```python
from build123d import *

# Parameters (mm, degrees)
F1_DEPTH = 40.2336
F0_R     = 10.16
F2_DEPTH = 15.7734
F3_SIZE  = 3.302


with BuildPart() as f1:
    # F0 (on Top) → F1 (new body)
    with BuildSketch(Plane.XY):
        with BuildLine():
            ThreePointArc((5.050141, -28.125197), (21.918467, -18.333342), (28.575, 0))
            ThreePointArc((28.575, 0), (21.918467, 18.333342), (5.050141, 28.125197))
            ThreePointArc((5.050141, 28.125197), (-28.575, 0), (5.050141, -28.125197))
        make_face()
        with BuildLine():
            ThreePointArc((13.447765, -4.826), (-14.2875, 0), (13.447765, 4.826))
            Line((13.447765, 4.826), (18.5293, 4.826))
            Line((18.5293, 4.826), (18.5293, -4.826))
            Line((18.5293, -4.826), (13.447765, -4.826))
        make_face(mode=Mode.SUBTRACT)
    extrude(amount=F1_DEPTH)

    # F0 (on Top) → F2 (join)
    with BuildSketch(Plane.XY):
        with BuildLine():
            ThreePointArc((5.050141, 28.125197), (21.918467, 18.333342), (28.575, 0))
            ThreePointArc((28.575, 0), (21.918467, -18.333342), (5.050141, -28.125197))
            Line((5.050141, -28.125197), (57.261665, -18.750131))
            ThreePointArc((57.261665, -18.750131), (72.944904, 0), (57.261665, 18.750131))
            Line((57.261665, 18.750131), (5.050141, 28.125197))
        make_face()
        with Locations((53.975, 0)):
            Circle(F0_R, mode=Mode.SUBTRACT)
    extrude(amount=F2_DEPTH)

    # F3
    f3_edges = [f1.edges().sort_by_distance(p)[0] for p in [
        (-5.050141, 28.125197, 40.2336),
    ]]
    chamfer(f3_edges, length=F3_SIZE)


solid = f1.part
```
Could you check a few things on this model? Use its own coordinates, in mm. A direction names the side the tool comes from. Round coordinates to 2 decimals unless told otherwise and drop trailing zeros. Write each loop counter-clockwise with the first axis right and the second up, starting at its lowest first coordinate (ties: lowest second). Pieces come first, ordered by that corner, then holes. Notation, with made-up numbers: M -34.75,-4 L 24.25,-4 A8 ccw 24.25,10 Z; hole C 5,-1 d4. An arc over 180 degrees is marked long. Answer in a Markdown table with one row per item. Add a question column.
Q1. Imagine slicing it at A-A (x = 0). Please give me the cut outline in (y, z) (1 decimal), then the cut area to 3 significant figures.
Q2. If I drill on line 1 (X direction, y = 0, z = 30.5) (1 decimal); line 2 (Z direction, x = 44, y = -14); line 3 (Y direction, x = 0, z = 24) (1 decimal), over which ranges is the centre line in solid material (lowest first)? Write a range as from..to.
Q3. Imagine slicing it at D-D (x = 63). Please give me the cut outline in (y, z).
Q4. Imagine slicing it at C-C (z = 3.5). Give the number of separate pieces and of enclosed holes in the cut face, then the cut area to 3 significant figures.
Q5. On a 3-axis mill with a long thin cutter (end or side, diameter ignored), from which of +Z, -Z, +X, -X, +Y, -Y can I reach the whole of each face in a straight line? I mean faces 1 (the flat face through (16, -4.826, 20)), 2 (the flat face through (21, 0, 0)). Say none if no direction works.
Q6. If we mould it in two halves opening along X, with no side actions, what happens to faces 3 (the flat face through (18.529, 0, 20)), 4 (the flat face through (11, -11, 40.234)), 5 (the cylindrical face through (72.94, -0.37, 7.78))? For each: +X half, -X half, draft (parallel to the pull), parting line (faces both ways), or undercut.
Q7. Will these pins go through, and if not, where does the flat tip stop? pin 1 Ø10.5 at (y, z) = (0.5, 13.5) entering from -X (3 decimals); pin 2 Ø5 at (y, z) = (10, 8.5) entering from -X; pin 3 Ø3 at (y, z) = (-19, 30.5) entering from +X.
Values:
| question | item | result |
|---|---|---|
| 1 | outline | M -28.6,0 L -14.3,0 L -14.3,40.2 L -25.3,40.2 L -28.6,36.9 Z; M 14.3,0 L 28.6,0 L 28.6,36.9 L 25.3,40.2 L 14.3,40.2 Z |
| 1 | area | 1,140 mm^2 |
| 2 | line 1 | -28.6..-14.3, 18.5..28.6 |
| 2 | line 2 | 0..15.77 |
| 2 | line 3 | -28.6..-14.3, 14.3..28.6 |
| 3 | outline | M -16.73,0 L -4.67,0 L -4.67,15.77 L -16.73,15.77 Z; M 4.67,0 L 16.73,0 L 16.73,15.77 L 4.67,15.77 Z |
| 4 | separate pieces | 1 |
| 4 | enclosed holes | 2 |
| 4 | area | 3,450 mm^2 |
| 5 | face 1 | +Z, -Z |
| 5 | face 2 | -Z, +X, -X, +Y, -Y |
| 6 | face 3 | undercut |
| 6 | face 4 | draft |
| 6 | face 5 | +X half |
| 7 | pin 1 | x = -28.575 |
| 7 | pin 2 | x = -27.57 |
| 7 | pin 3 | x = 22.59 |
